Model file for the job. Use its own axes, mm. Face numbers are marked on the shaded views. A direction names the side the tool comes from. Give positions to 0.01 mm unless a question says otherwise; leave off trailing zeros. Order: outer loops, then holes, each group sorted by start corner. A loop starts at its lowest first (then second) coordinate and runs counter-clockwise, first axis right, second up. Notation, with made-up numbers: (-23, -16) - (18, -16) arc R25 ccw to (18, 15) - close; hole circle Ø11 at (-20, -16). An arc over 180 degrees is marked (long way). Use CSV: the item, a comma, the result in double quotes. Start each with the question number.
(1) Pull direction Z, two halves, no side cores. Call the marked faces 1, 2, 3 and 4: +Z half, -Z half, draft (parallel to the pull), parting line (faces both ways), or undercut.
(2) Band-saw the part on D-D, the plane y = -6.5. Give the cut face in (x, z), then the cut area to 3 significant figures.
(3) Band-saw the part on A-A, the plane z = -18. Give the cut face in (x, y), then the cut area to 3 significant figures.
(4) Band-saw the part on C-C, the plane z = -48. Give the cut face in (x, y).
(5) Band-saw the part on B-B, the plane x = -49. Give the cut face in (y, z).
(6) Probe L1, parallel to Y at x = -78, z = -37; L2, parallel to X at y = -4, z = -23; L3, parallel to Y at x = -51, z = -41.5. List the from-to ranges inside material, lowest first.
(7) Drop flat-ended pins along their axis: pin 1 Ø3.5 at (y, z) = (-1.5, -32.5) entering from +X; pin 2 Ø1.6 at (x, z) = (-54.5, -26.5) entering from -Y; pin 3 Ø2 at (y, z) = (-12, -20.5) entering from -X. Give the stop position or say it passes through.
(8) Tool access for the marked faces 5, 6 and 7: list every direction of +Z, -Z, +X, -X, +Y, -Y with a clear straight run to the whole face (end or side of a thin tool).
from build123d import *

# Parameters (mm, degrees)
SKETCH4_R           = 2.5
BOSS_EXTRUDE1_DEPTH = 3
SKETCH5_W           = 3
SKETCH5_H           = 44.34
BOSS_EXTRUDE2_DEPTH = 34
SKETCH11_R          = 1
BOSS_EXTRUDE3_DEPTH = 3
RIB7_REACH          = 99.577
SKETCH15_WALL_W     = 207.051776086
SKETCH15_WALL_H     = 2
LPATTERN2_COUNT     = 3
LPATTERN2_PITCH     = 4
LPATTERN2_COL_COUNT = 3
LPATTERN2_COL_PITCH = 4
RIB8_REACH          = 107.913
SKETCH16_WALL_W     = 219.851918098
SKETCH16_WALL_H     = 10
FILLET3_R           = 1
SKETCH17_W          = 24.34
SKETCH17_H          = 7
CUT_EXTRUDE1_DEPTH  = 2
FILLET4_R           = 0.5


with BuildPart() as part:
    # Sketch4 → Boss-Extrude1 (new body)
    with BuildSketch(Plane(origin=(0, 0, 0), x_dir=(1, 0, 0), z_dir=(0, 1, 0))):
        with BuildLine():
            Line((-61.549656869, 55.367306066), (-61.549656869, 1.027306066))
            Line((-61.549656869, 1.027306066), (-50.119656869, 1.027306066))
            ThreePointArc((-50.119656869, 1.027306066), (-41.999656869, 9.147306066), (-50.119656869, 17.267306066))
            Line((-50.119656869, 17.267306066), (-50.119656869, 39.127306066))
            ThreePointArc((-50.119656869, 39.127306066), (-41.999656869, 47.247306066), (-50.119656869, 55.367306066))
            Line((-50.119656869, 55.367306066), (-61.549656869, 55.367306066))
        make_face()
        with Locations(Location((-50.119656869, 47.247306066, 0), (0, 0, 270))):
            Circle(SKETCH4_R, mode=Mode.SUBTRACT)
        with Locations(Location((-50.119656869, 9.147306066, 0), (0, 0, 270))):
            Circle(SKETCH4_R, mode=Mode.SUBTRACT)
    extrude(amount=-BOSS_EXTRUDE1_DEPTH)

    # Sketch5 → Boss-Extrude2 (add)
    with BuildSketch(Plane.XZ.offset(3)):
        with Locations((-60.049656869, -28.197306066)):
            Rectangle(SKETCH5_W, SKETCH5_H)
    extrude(amount=BOSS_EXTRUDE2_DEPTH)

    # Sketch11 → Boss-Extrude3 (add)
    with BuildSketch(Plane.XZ.offset(37)):
        Polygon((-86.105180159, -35.362306066), (-86.105180159, -50.367306066), (-61.549656869, -50.367306066), (-61.549656869, -6.027306066), (-86.105180159, -6.027306066), (-86.105180159, -11.592306066), (-73.855180159, -11.592306066), (-73.855180159, -35.362306066), align=None)
        with Locations(Location((-83.485180159, -37.742306066, 0), (0, 0, 270))):
            Circle(SKETCH11_R, mode=Mode.SUBTRACT)
        with Locations(Location((-79.985180159, -37.742306066, 0), (0, 0, 270))):
            Circle(SKETCH11_R, mode=Mode.SUBTRACT)
        with Locations(Location((-76.485180159, -37.742306066, 0), (0, 0, 270))):
            Circle(SKETCH11_R, mode=Mode.SUBTRACT)
        with Locations(Location((-83.485180159, -9.212306066, 0), (0, 0, 270))):
            Circle(SKETCH11_R, mode=Mode.SUBTRACT)
        with Locations(Location((-79.985180159, -9.212306066, 0), (0, 0, 270))):
            Circle(SKETCH11_R, mode=Mode.SUBTRACT)
        with Locations(Location((-76.485180159, -9.212306066, 0), (0, 0, 270))):
            Circle(SKETCH11_R, mode=Mode.SUBTRACT)
    extrude(amount=-BOSS_EXTRUDE3_DEPTH)

    # Sketch15 wall → Rib7 (add, up to next)
    with BuildSketch(Plane(origin=(-54.334656869, -5.592920769, -28.197306066), x_dir=(0.851741772014, 0.523961786591, 0), z_dir=(-0.523961786591, 0.851741772014, 0)), mode=Mode.PRIVATE) as rib7_sk1:
        Rectangle(SKETCH15_WALL_W, SKETCH15_WALL_H)
    rib7_tool1 = extrude(rib7_sk1.sketch, amount=RIB7_REACH, mode=Mode.PRIVATE) - part.part
    rib7 = rib7_tool1.solids().sort_by_distance((-54.334656869, -5.592920769, -28.197306066))[0]
    add(rib7)

    # LPattern2: Rib7 ×3
    with Locations(*[(0, 0, -i * LPATTERN2_PITCH) for i in range(1, LPATTERN2_COUNT)]):
        add(rib7)

    # LPattern2 col: Rib7 ×3
    with Locations(*[(0, 0, i * LPATTERN2_COL_PITCH) for i in range(1, LPATTERN2_COL_COUNT)]):
        add(rib7)

    # Sketch16 wall → Rib8 (add, up to next)
    with BuildSketch(Plane(origin=(-63.680227165, -31.869429704, -6.027306066), x_dir=(0.707106781187, 0.707106781187, 0), z_dir=(-0.707106781187, 0.707106781187, 0)), mode=Mode.PRIVATE) as rib8_sk1:
        with Locations((0, 5)):
            Rectangle(SKETCH16_WALL_W, SKETCH16_WALL_H)
    rib8_tool1 = extrude(rib8_sk1.sketch, amount=-RIB8_REACH, mode=Mode.PRIVATE) - part.part
    rib8 = rib8_tool1.solids().sort_by_distance((-63.680227165, -31.869429704, -6.027306066))[0]
    add(rib8)

    # Mirror1: Rib8 across plane
    add(rib8.mirror(Plane.XY.offset(-28.197306066)))

    # Fillet3
    fillet3_edges = [part.edges().sort_by_distance(p)[0] for p in [
        (-61.549656869, -1.5, -1.027306066),
        (-61.549656869, -1.5, -55.367306066),
        (-60.049656869, -3, -50.367306066),
        (-60.049656869, -3, -6.027306066),
        (-58.549656869, -37, -28.197306066),
        (-86.105180159, -35.5, -11.592306066),
        (-86.105180159, -35.5, -6.027306066),
        (-86.105180159, -35.5, -50.367306066),
        (-86.105180159, -35.5, -35.362306066),
    ]]
    fillet(fillet3_edges, radius=FILLET3_R)

    # Sketch17 → Cut-Extrude1 (cut)
    with BuildSketch(Plane.ZY.offset(61.549656869)):
        with Locations((-28.197306066, -30.5)):
            Rectangle(SKETCH17_W, SKETCH17_H)
    extrude(amount=-CUT_EXTRUDE1_DEPTH, mode=Mode.SUBTRACT)

    # Fillet4
    fillet4_edges = [part.edges().sort_by_distance(p)[0] for p in [
        (-73.855180159, -35.5, -35.362306066),
        (-73.855180159, -35.5, -11.592306066),
    ]]
    fillet(fillet4_edges, radius=FILLET4_R)


solid = part.part
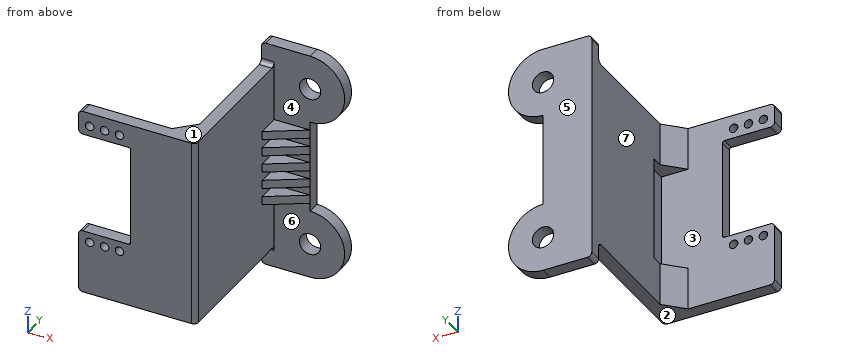
Answer block:
1,face 1,"+Z half"
1,face 2,"-Z half"
1,face 3,"undercut"
1,face 4,"draft"
2,outline,"(-61.55, -50.37) - (-58.55, -50.37) - (-58.55, -37.2) - (-55.81, -37.2) - (-55.81, -35.2) - (-58.55, -35.2) - (-58.55, -33.2) - (-55.81, -33.2) - (-55.81, -31.2) - (-58.55, -31.2) - (-58.55, -29.2) - (-55.81, -29.2) - (-55.81, -27.2) - (-58.55, -27.2) - (-58.55, -25.2) - (-55.81, -25.2) - (-55.81, -23.2) - (-58.55, -23.2) - (-58.55, -21.2) - (-55.81, -21.2) - (-55.81, -19.2) - (-58.55, -19.2) - (-58.55, -6.03) - (-61.55, -6.03) - close"
2,area,"160 mm2"
3,outline,"(-73.86, -37) - (-59.55, -37) arc R1 ccw to (-58.55, -36) - (-58.55, -3) - (-50.12, -3) - (-50.12, 0) - (-61.55, 0) - (-61.55, -27) - (-59.55, -27) - (-59.55, -34) - (-73.86, -34) - close"
3,area,"159 mm2"
4,outline,"(-86.11, -37) - (-59.55, -37) arc R1 ccw to (-58.55, -36) - (-58.55, -3) - (-52.5, -3) - (-52.5, 0) - (-61.55, 0) - (-61.55, -29.74) - (-65.81, -34) - (-86.11, -34) - close; (-47.74, -3) - (-42.03, -3) - (-42.03, 0) - (-47.74, 0) - close"
5,outline,"(-3, -55.29) - (0, -55.29) - (0, -49.48) - (-3, -49.48) - close; (-3, -45.01) - (0, -45.01) - (0, -39.2) - (-3, -39.2) - close; (-3, -17.19) - (0, -17.19) - (0, -11.38) - (-3, -11.38) - close; (-3, -6.91) - (0, -6.91) - (0, -1.1) - (-3, -1.1) - close"
6,L1,"y = -37 to -34"
6,L2,"x = -61.55 to -58.55"
6,L3,"y = -3 to 0"
7,pin 1,"stops at x = -50.12"
7,pin 2,"stops at y = -5.94"
7,pin 3,"stops at x = -61.55"
8,face 5,"+Z, -Z, +X, -X, +Y"
8,face 6,"-Z, +X, -Y"
8,face 7,"+Z, -Z, -X, +Y"
